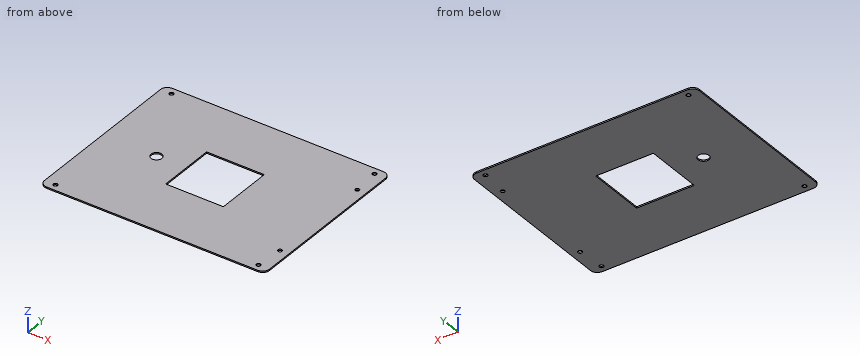
```python
from build123d import *

# Parameters (mm, degrees)
SKETCH_1_R          = 1.55
EXTRUDE_1_DEPTH     = 1
SKETCH_3_R          = 1.5
CUT_EXTRUDE_2_DEPTH = 10
SKETCH_4_R          = 4
CUT_EXTRUDE_3_DEPTH = 10
SKETCH_5_W          = 42.3
SKETCH_5_H          = 42.3
CUT_EXTRUDE_4_DEPTH = 10


with BuildPart() as part:
    # 草图1 → 凸台-拉伸1 (new body)
    with BuildSketch(Plane.XY):
        with BuildLine():
            Line((-77.5, 65), (77.5, 65))
            ThreePointArc((77.5, 65), (81.035533906, 63.535533906), (82.5, 60))
            Line((82.5, 60), (82.5, -60))
            ThreePointArc((82.5, -60), (81.035533906, -63.535533906), (77.5, -65))
            Line((77.5, -65), (-77.5, -65))
            ThreePointArc((-77.5, -65), (-81.035533906, -63.535533906), (-82.5, -60))
            Line((-82.5, -60), (-82.5, 60))
            ThreePointArc((-82.5, 60), (-81.035533906, 63.535533906), (-77.5, 65))
        make_face()
        with Locations((-74.5, 60)):
            Circle(SKETCH_1_R, mode=Mode.SUBTRACT)
        with Locations((74.5, 60)):
            Circle(SKETCH_1_R, mode=Mode.SUBTRACT)
        with Locations((74.5, -60)):
            Circle(SKETCH_1_R, mode=Mode.SUBTRACT)
        with Locations((-74.5, -60)):
            Circle(SKETCH_1_R, mode=Mode.SUBTRACT)
    extrude(amount=EXTRUDE_1_DEPTH)

    # 草图3 → 切除-拉伸2 (cut)
    with BuildSketch(Plane.XY.offset(1)):
        with Locations((76, 40)):
            Circle(SKETCH_3_R)
        with Locations((76, -40)):
            Circle(SKETCH_3_R)
    extrude(amount=-CUT_EXTRUDE_2_DEPTH, mode=Mode.SUBTRACT)

    # 草图4 → 切除-拉伸3 (cut)
    with BuildSketch(Plane.XY.offset(1)):
        with Locations((-42.951152845, 0)):
            Circle(SKETCH_4_R)
    extrude(amount=-CUT_EXTRUDE_3_DEPTH, mode=Mode.SUBTRACT)

    # 草图5 → 切除-拉伸4 (cut)
    with BuildSketch(Plane.XY.offset(1)):
        Rectangle(SKETCH_5_W, SKETCH_5_H)
    extrude(amount=-CUT_EXTRUDE_4_DEPTH, mode=Mode.SUBTRACT)


solid = part.part
```
For this review, take the finished solid that the model builds, in its own axes (mm). Coordinates: 2 decimals unless noted, no trailing zeros. Write each loop counter-clockwise with the first axis right and the second up, starting at its lowest first coordinate (ties: lowest second). Pieces come first, ordered by that corner, then holes.
(1) Wall thickness on probe 1 along Y at (x, z) = (-74.5, 0.65); probe 2 along Y at (x, z) = (-42.5, 0.4); probe 3 along X at (y, z) = (-19.5, 0.65): over which ranges is each line inside the solid? List them lowest first.
(2) Add section C-C on x = 3. Give the boundary of the cut face in (y, z).
(3) For pin 1 Ø2.5 at (x, y) = (-74.5, -60) entering from -Z; pin 2 Ø1.5 at (x, y) = (15, -29.5) entering from -Z, all flat-tipped, find the tip position at first contact; note any pin that passes through.
(4) Add section B-B on z = 0.5. Count the separate pieces of the cut face and the enclosed holes in it, then the cut area to 3 significant figures.
(5) Add section A-A on y = -7. Give the boundary of the cut face in (x, z), then the cut area to 3 significant figures.
Answer sheet:
1. probe 1: y = -65 to -61.55, -58.45 to 58.45, 61.55 to 65
1. probe 2: y = -65 to -3.97, 3.97 to 65
1. probe 3: x = -82.5 to -21.15, 21.15 to 82.5
2. outline: (-65, 0) - (-21.15, 0) - (-21.15, 1) - (-65, 1) - close; (21.15, 0) - (65, 0) - (65, 1) - (21.15, 1) - close
3. pin 1: passes through
3. pin 2: stops at z = 0
4. separate pieces: 1
4. enclosed holes: 8
4. area: 19,500 mm2
5. outline: (-82.5, 0) - (-21.15, 0) - (-21.15, 1) - (-82.5, 1) - close; (21.15, 0) - (82.5, 0) - (82.5, 1) - (21.15, 1) - close
5. area: 123 mm2
